Check sheet for the modelled part. Datum: model origin and axes. Units: mm. A direction names the side the tool comes from. Give positions to 0.01 mm unless a question says otherwise; leave off trailing zeros. Order: outer loops, then holes, each group sorted by start corner. A loop starts at its lowest first (then second) coordinate and runs counter-clockwise, first axis right, second up.
from build123d import *

# Parameters (mm, degrees)
F0_W      = 440
F0_H      = 250
F1_DEPTH  = 5
F2_W      = 250
F2_H      = 200
F2_W_2    = 350
F2_H_2    = 250
F3_DEPTH  = 5
F4_R      = 150
F5_R      = 100
F6_R      = 49.99999
F7_SIZE2  = 150
F7_SIZE   = 50
F8_SIZE2  = 50
F8_SIZE   = 150
F10_DEPTH = 25


# Not quite as in the source:
# - a fillet or chamfer is up to 0.001 mm smaller than in the source, because OpenCascade refuses the exact size


with BuildPart() as f1:
    # F0 (on Top) → F1 (new body)
    with BuildSketch(Plane.XY):
        Rectangle(F0_W, F0_H)
    extrude(amount=F1_DEPTH)

    # F2 (on face) → F3 (join)
    with BuildSketch(Plane(origin=(0, 0, 0), x_dir=(1, 0, 0), z_dir=(0, 0, -1))):
        with Locations((-295, 175)):
            Rectangle(F2_W, F2_H)
        with Locations((295, 175)):
            Rectangle(F2_W, F2_H)
        with Locations((-245, -200)):
            Rectangle(F2_W_2, F2_H_2)
        with Locations((245, -200)):
            Rectangle(F2_W_2, F2_H_2)
    extrude(amount=-F3_DEPTH)

    # F4
    f4_edges = [f1.edges().sort_by_distance(p)[0] for p in [
        (-420, -275, 2.5),
        (420, -275, 2.5),
    ]]
    fillet(f4_edges, radius=F4_R)

    # F5
    f5_edges = [f1.edges().sort_by_distance(p)[0] for p in [
        (170, -125, 2.5),
        (-170, -125, 2.5),
    ]]
    fillet(f5_edges, radius=F5_R)

    # F6 (radius 50 in the source; OpenCascade refuses exactly that, so slightly less here)
    f6_edges = [f1.edges().sort_by_distance(p)[0] for p in [
        (-170, -275, 2.5),
        (170, -275, 2.5),
    ]]
    fillet(f6_edges, radius=F6_R)

    # F7
    f7_edges = [f1.edges().sort_by_distance(p)[0] for p in [
        (420, 325, 2.5),
    ]]
    f7_side = f1.faces().sort_by_distance((245, 325, 2.5))[0]
    chamfer(f7_edges, length=F7_SIZE, length2=F7_SIZE2, reference=f7_side)

    # F8
    f8_edges = [f1.edges().sort_by_distance(p)[0] for p in [
        (-420, 325, 2.5),
    ]]
    f8_side = f1.faces().sort_by_distance((-420, 200, 2.5))[0]
    chamfer(f8_edges, length=F8_SIZE, length2=F8_SIZE2, reference=f8_side)

    # F9 (on face) → F10 (cut)
    with BuildSketch(Plane.XY.offset(5)):
        Polygon((-220, 325), (-70, 125), (-70, 325), align=None)
        Polygon((70, 325), (70, 125), (220, 325), align=None)
    extrude(amount=-F10_DEPTH, mode=Mode.SUBTRACT)


solid = f1.part
1) Depth check by flat-ended pin: pin 1 Ø2.5 at (x, z) = (-353, 2.5) entering from -Y; pin 2 Ø2 at (y, z) = (-32.5, 2) entering from +X; pin 3 Ø2.5 at (x, z) = (15.5, 1.5) entering from +Y. Enter the tip coordinate at first touch or a pass-through.
Recorded:
pin 1: stops at y = -250.77
pin 2: stops at x = 220
pin 3: stops at y = 125
2) Material ranges on L1, parallel to Y at x = -271.5, z = 0.95; L2, parallel to X at y = 17, z = 4.5; L3, parallel to X at y = -188, z = 0.45, recorded low to high.
Recorded:
L1: y = -274.99 to -75, 75 to 325
L2: x = -220 to 220
L3: x = -406.13 to -162.9, 162.9 to 406.13
3) Draft check along X on faces 1 (the face through (143.95, 223.6, 2.54)), 2 (the face through (-377.23, -229.89, 2.54)), 3 (the face through (374.89, -232.23, 2.54)). Enter one of: +X half, -X half, draft (parallel to the pull), parting line (faces both ways), or undercut.
Recorded:
face 1: undercut
face 2: -X half
face 3: +X half
4) Section check B-B, the plane x = -243. Record the cut outline in (y, z), then the cut area to 3 significant figures.
Recorded:
outline: (-275, 0) - (-75, 0) - (-75, 5) - (-275, 5) - close; (75, 0) - (325, 0) - (325, 5) - (75, 5) - close
area: 2,250 mm2
5) Set-up check for faces 4 (the face through (395.35, 248.95, 2.47)), 5 (the face through (-146.05, 226.4, 2.54)), 6 (the face through (-184.258, -259.964, 2.535)): record each of +Z, -Z, +X, -X, +Y, -Y from which the full face is reachable in a straight line by a thin tool's end or side.
Recorded:
face 4: +Z, -Z, +X, +Y
face 5: +Z, -Z, +Y
face 6: +Z, -Z, -Y
6) Section check A-A, the plane y = 220. Record the cut outline in (x, z).
Recorded:
outline: (-405, 0) - (-141.25, 0) - (-141.25, 5) - (-405, 5) - close; (141.25, 0) - (405, 0) - (405, 5) - (141.25, 5) - close
7) Section check D-D, the plane y = -3.5. Record the cut outline in (x, z).
Recorded:
outline: (-220, 0) - (220, 0) - (220, 5) - (-220, 5) - close
